Source: CAD feature listing. Evaluate the final solid. Frame: model axes, mm. A direction names the side the tool comes from. Round coordinates to 2 decimals unless told otherwise and drop trailing zeros. Order: outer loops, then holes, each group sorted by start corner. A loop starts at its lowest first (then second) coordinate and runs counter-clockwise, first axis right, second up. Notation, with made-up numbers: M 9,-28.5 L 68,-28.5 A23 cw 68,-11.5 Z; hole C 75,17.25 d3. An arc over 180 degrees is marked long. Use one line per item in the form item = value. Start each with the question number.
Q1. Section B-B (x = 0). Return the cut outline in (y, z), plus the area to 3 significant figures.
Q2. Section D-D (y = -36.5). Return the cut outline in (x, z).
Q3. Section C-C (y = -110.5). Return the cut outline in (x, z).
Q4. Reachability of faces 1 (the flat face through (16, 0, 1)), 2 (the cylindrical face through (-31.37, -135.05, 1.38)) from +Z, -Z, +X, -X, +Y, -Y: full face, straight path, thin tool, end or side. Return the list, or none.
Q5. Section A-A (z = 0). Return the cut outline in (x, y), plus the area to 3 significant figures.
Q6. Contact query for flat-ended pins moving along their axis: pin 1 (10 mm diameter, centred on x = 25.5, z = -55.5, fed in from -Y); pin 2 (6 mm diameter, centred on y = -58, z = 56.5, fed in from +X); pin 3 (4 mm diameter, centred on y = -69.5, z = -37, fed in from +X). Output: stop coordinate, or through.
Q7. Material intervals for probe 1 along Z at (x, y) = (0, -100); probe 2 along Z at (x, y) = (0, -49); probe 3 along Y at (x, z) = (-45, 35.5), sorted ascending.
from build123d import *

# Parameters (mm, degrees)
F0_R      = 75
F1_DEPTH  = 76.2
F2_R      = 31.399649
F3_DEPTH  = 127
F3_FACE_R = 31.399649
F4_R      = 15.247419
F5_DEPTH  = 331.978
F6_R      = 7.62
F7_R      = 7.62


with BuildPart() as f1:
    # F0 (on Front) → F1 (new body)
    with BuildSketch(Plane.XZ):
        Circle(F0_R)
    extrude(amount=F1_DEPTH)

    # F2 (on face) → F3 (join)
    with BuildSketch(Plane.XZ.offset(76.2)):
        Circle(F2_R)
    extrude(amount=F3_DEPTH)

    # F3_face (on face) + F4 (on Front) → F5 (cut)
    with BuildSketch(Plane.XZ.offset(203.2)):
        Circle(F3_FACE_R)
    with BuildSketch(Plane.XZ):
        Circle(F4_R)
    extrude(amount=F5_DEPTH, mode=Mode.SUBTRACT)

    # F6
    f6_edges = [f1.edges().sort_by_distance(p)[0] for p in [
        (-31.399649, -203.2, 0),
    ]]
    fillet(f6_edges, radius=F6_R)

    # F7
    f7_edges = [f1.edges().sort_by_distance(p)[0] for p in [
        (-75, -76.2, 0),
    ]]
    fillet(f7_edges, radius=F7_R)


solid = f1.part
Results list:
q1.outline = M -203.2,-23.78 A7.62 ccw -195.58,-31.4 L -76.2,-31.4 L -76.2,-67.38 A7.62 ccw -68.58,-75 L 0,-75 L 0,-15.25 L -203.2,-15.25 Z; M -203.2,15.25 L 0,15.25 L 0,75 L -68.58,75 A7.62 ccw -76.2,67.38 L -76.2,31.4 L -195.58,31.4 A7.62 ccw -203.2,23.78 Z
q1.area = 13,200 mm2
q2.outline = C 0,0 d150; hole C 0,0 d30.49
q3.outline = C 0,0 d62.8; hole C 0,0 d30.49
q4.face_1 = +Z, -Z, +X, -X, +Y
q4.face_2 = -Y
q5.outline = M -75,-68.58 A7.62 ccw -67.38,-76.2 L -31.4,-76.2 L -31.4,-195.58 A7.62 ccw -23.78,-203.2 L -15.25,-203.2 L -15.25,0 L -75,0 Z; M 15.25,-203.2 L 23.78,-203.2 A7.62 ccw 31.4,-195.58 L 31.4,-76.2 L 67.38,-76.2 A7.62 ccw 75,-68.58 L 75,0 L 15.25,0 Z
q5.area = 13,200 mm2
q6.pin_1 = -76.2
q6.pin_2 = 52.56
q6.pin_3 = 66.29
q7.probe_1 = -31.4 to -15.25, 15.25 to 31.4
q7.probe_2 = -75 to -15.25, 15.25 to 75
q7.probe_3 = -76.2 to 0
